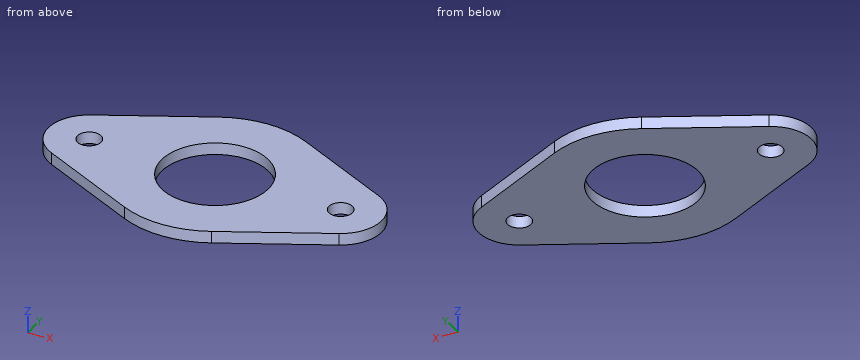
from build123d import *

# Parameters (mm, degrees)
F0_R     = 4
F0_R_2   = 18
F1_DEPTH = 2


with BuildPart() as f1:
    # F0 (on Top) → F1 (new body, symmetric)
    with BuildSketch(Plane.XY):
        with BuildLine():
            ThreePointArc((-31.732280933, 8.5683694007), (-39.5639115572, 13.473057404), (-48.7344588715, 12.3366311636))
            ThreePointArc((-48.7344588715, 12.3366311636), (-56.35, 0), (-48.7344588715, -12.3366311636))
            ThreePointArc((-48.7344588715, -12.3366311636), (-39.5639115572, -13.473057404), (-31.732280933, -8.5683694007))
            ThreePointArc((-31.732280933, -8.5683694007), (-32.8687481872, 0), (-31.732280933, 8.5683694007))
        make_face()
        with Locations((-42.55, 0)):
            Circle(F0_R, mode=Mode.SUBTRACT)
        with BuildLine():
            ThreePointArc((-28.75, 0), (-29.5168782879, 4.5362692201), (-31.732280933, 8.5683694007))
            ThreePointArc((-31.732280933, 8.5683694007), (-32.8687481872, 0), (-31.732280933, -8.5683694007))
            ThreePointArc((-31.732280933, -8.5683694007), (-29.5168782879, -4.5362692201), (-28.75, 0))
        make_face()
        with BuildLine():
            ThreePointArc((14.7301029944, 29.3833060286), (0, 32.8687481872), (-14.7301029944, 29.3833060286))
            ThreePointArc((-14.7301029944, 29.3833060286), (-25.455916341, 20.7930500561), (-31.732280933, 8.5683694007))
            ThreePointArc((-31.732280933, 8.5683694007), (-29.5168782879, 4.5362692201), (-28.75, 0))
            ThreePointArc((-28.75, 0), (-29.5168782879, -4.5362692201), (-31.732280933, -8.5683694007))
            ThreePointArc((-31.732280933, -8.5683694007), (-25.455916341, -20.7930500561), (-14.7301029944, -29.3833060286))
            ThreePointArc((-14.7301029944, -29.3833060286), (0, -32.8687481872), (14.7301029944, -29.3833060286))
            ThreePointArc((14.7301029944, -29.3833060286), (25.455916341, -20.7930500561), (31.732280933, -8.5683694007))
            ThreePointArc((31.732280933, -8.5683694007), (28.75, 0), (31.732280933, 8.5683694007))
            ThreePointArc((31.732280933, 8.5683694007), (25.455916341, 20.7930500561), (14.7301029944, 29.3833060286))
        make_face()
        Circle(F0_R_2, mode=Mode.SUBTRACT)
        with BuildLine():
            Line((-14.7301029944, 29.3833060286), (-48.7344588715, 12.3366311636))
            ThreePointArc((-48.7344588715, 12.3366311636), (-39.5639115572, 13.473057404), (-31.732280933, 8.5683694007))
            ThreePointArc((-31.732280933, 8.5683694007), (-25.455916341, 20.7930500561), (-14.7301029944, 29.3833060286))
        make_face()
        with BuildLine():
            ThreePointArc((-31.732280933, -8.5683694007), (-39.5639115572, -13.473057404), (-48.7344588715, -12.3366311636))
            Line((-48.7344588715, -12.3366311636), (-14.7301029944, -29.3833060286))
            ThreePointArc((-14.7301029944, -29.3833060286), (-25.455916341, -20.7930500561), (-31.732280933, -8.5683694007))
        make_face()
        with BuildLine():
            ThreePointArc((32.8687481872, 0), (32.5833926931, 4.3217042936), (31.732280933, 8.5683694007))
            ThreePointArc((31.732280933, 8.5683694007), (28.75, 0), (31.732280933, -8.5683694007))
            ThreePointArc((31.732280933, -8.5683694007), (32.5833926931, -4.3217042936), (32.8687481872, 0))
        make_face()
        with BuildLine():
            ThreePointArc((31.732280933, -8.5683694007), (25.455916341, -20.7930500561), (14.7301029944, -29.3833060286))
            Line((14.7301029944, -29.3833060286), (48.7344588715, -12.3366311636))
            ThreePointArc((48.7344588715, -12.3366311636), (39.5639115572, -13.473057404), (31.732280933, -8.5683694007))
        make_face()
        with BuildLine():
            ThreePointArc((48.7344588715, 12.3366311636), (39.5639115572, 13.473057404), (31.732280933, 8.5683694007))
            ThreePointArc((31.732280933, 8.5683694007), (32.5833926931, 4.3217042936), (32.8687481872, 0))
            ThreePointArc((32.8687481872, 0), (32.5833926931, -4.3217042936), (31.732280933, -8.5683694007))
            ThreePointArc((31.732280933, -8.5683694007), (39.5639115572, -13.473057404), (48.7344588715, -12.3366311636))
            ThreePointArc((48.7344588715, -12.3366311636), (54.2927750644, -7.2489470812), (56.35, 0))
            ThreePointArc((56.35, 0), (54.2927750644, 7.2489470812), (48.7344588715, 12.3366311636))
        make_face()
        with Locations((42.55, 0)):
            Circle(F0_R, mode=Mode.SUBTRACT)
        with BuildLine():
            Line((48.7344588715, 12.3366311636), (14.7301029944, 29.3833060286))
            ThreePointArc((14.7301029944, 29.3833060286), (25.455916341, 20.7930500561), (31.732280933, 8.5683694007))
            ThreePointArc((31.732280933, 8.5683694007), (39.5639115572, 13.473057404), (48.7344588715, 12.3366311636))
        make_face()
    extrude(amount=F1_DEPTH, both=True)


solid = f1.part
Verification items for the finished model (mm, model axes). Coordinates: 2 decimals unless noted, no trailing zeros. Write each loop counter-clockwise with the first axis right and the second up, starting at its lowest first coordinate (ties: lowest second). Pieces come first, ordered by that corner, then holes. Notation, with made-up numbers: M -4.75,12.5 L 31.25,12.5 A30 cw 31.25,47.5 Z; hole C 43,-5.5 d4. An arc over 180 degrees is marked long. Use a Markdown table: item, result.
Q1. Sectioned sample at C-C, the plane z = -0.4. Record the boundary of the cut face in (x, y).
Reply:
| item | result |
|---|---|
| outline | M -48.73,-12.34 L -14.73,-29.38 A32.87 ccw 14.73,-29.38 L 48.73,-12.34 A13.8 ccw 48.73,12.34 L 14.73,29.38 A32.87 ccw -14.73,29.38 L -48.73,12.34 A13.8 ccw Z; hole C -42.55,0 d8; hole C 0,0 d36; hole C 42.55,0 d8 |
Q2. Sectioned sample at B-B, the plane x = 0. Record the boundary of the cut face in (y, z), plus the area to 3 significant figures.
Reply:
| item | result |
|---|---|
| outline | M -32.87,-2 L -18,-2 L -18,2 L -32.87,2 Z; M 18,-2 L 32.87,-2 L 32.87,2 L 18,2 Z |
| area | 119 mm² |
Q3. Sectioned sample at D-D, the plane y = 10.5. Record the boundary of the cut face in (x, z).
Reply:
| item | result |
|---|---|
| outline | M -51.5,-2 L -14.62,-2 L -14.62,2 L -51.5,2 Z; M 14.62,-2 L 51.5,-2 L 51.5,2 L 14.62,2 Z |
Q4. Sectioned sample at A-A, the plane y = 0. Record the boundary of the cut face in (x, z), plus the area to 3 significant figures.
Reply:
| item | result |
|---|---|
| outline | M -56.35,-2 L -46.55,-2 L -46.55,2 L -56.35,2 Z; M -38.55,-2 L -18,-2 L -18,2 L -38.55,2 Z; M 18,-2 L 38.55,-2 L 38.55,2 L 18,2 Z; M 46.55,-2 L 56.35,-2 L 56.35,2 L 46.55,2 Z |
| area | 243 mm² |
Q5. Thickness scan on line 1 (Y direction, x = 0, z = 0.8); line 2 (Y direction, x = 42.55, z = -0.25); line 3 (X direction, y = 9.5, z = -0.5). Record the ranges inside material, lowest first.
Reply:
| item | result |
|---|---|
| line 1 | y = -32.87 to -18, 18 to 32.87 |
| line 2 | y = -15.44 to -4, 4 to 15.44 |
| line 3 | x = -52.56 to -15.29, 15.29 to 52.56 |
Q6. Go/stop test with flat-tipped pins: P1, Ø6.5, axis at x = 42.55, y = 0, coming from the -Z side; P2, Ø1, axis at x = -45, z = -1, coming from the +Y side; P3, Ø2, axis at x = 24.5, z = -0.5, coming from the +Y side; P4, Ø1, axis at x = -39.5, z = 0, coming from the +Y side. Record where each tip stops, or that it passes through.
Reply:
| item | result |
|---|---|
| P1 | passes through |
| P2 | stops at y = 14.46 |
| P3 | stops at y = 24.99 |
| P4 | stops at y = 17.22 |
